```python
from build123d import *

# Parameters (mm, degrees)
F0_W     = 300
F0_H     = 24.5
F0_R     = 2.65
F1_DEPTH = 2
F2_DEPTH = 10
F3_DEPTH = 30
F4_R     = 1.7
F5_DEPTH = 2
F6_R     = 1.25
F7_DEPTH = 2


with BuildPart() as f1:
    # F0 (on Top) → F1 (new body)
    with BuildSketch(Plane.XY):
        Rectangle(F0_W, F0_H)
        with Locations((-60, 0)):
            Circle(F0_R, mode=Mode.SUBTRACT)
        with Locations((-45, 0)):
            Circle(F0_R, mode=Mode.SUBTRACT)
        with Locations((-30, 0)):
            Circle(F0_R, mode=Mode.SUBTRACT)
        with Locations((-15, 0)):
            Circle(F0_R, mode=Mode.SUBTRACT)
        Circle(F0_R, mode=Mode.SUBTRACT)
        with Locations((15, 0)):
            Circle(F0_R, mode=Mode.SUBTRACT)
        with Locations((30, 0)):
            Circle(F0_R, mode=Mode.SUBTRACT)
        with Locations((45, 0)):
            Circle(F0_R, mode=Mode.SUBTRACT)
        with Locations((60, 0)):
            Circle(F0_R, mode=Mode.SUBTRACT)
    extrude(amount=F1_DEPTH)

    # F2 (add): a face of the model
    f2_faces = [f1.faces().sort_by_distance(p)[0] for p in [
        (-150, 0, 1),
    ]]
    extrude(f2_faces, amount=F2_DEPTH)

    # F3 (add): a face of the model
    f3_faces = [f1.faces().sort_by_distance(p)[0] for p in [
        (150, 0, 1),
    ]]
    extrude(f3_faces, amount=F3_DEPTH)

    # F4 (on face) → F5 (cut, through all)
    with BuildSketch(Plane.XY.offset(2)):
        with Locations((-153.6, 0)):
            Circle(F4_R)
    extrude(amount=-F5_DEPTH, mode=Mode.SUBTRACT)

    # F6 (on face) → F7 (cut, through all)
    with BuildSketch(Plane.XY.offset(2)):
        with Locations((158.75, -7.25)):
            Circle(F6_R)
    extrude(amount=-F7_DEPTH, mode=Mode.SUBTRACT)


solid = f1.part
```
Source: CAD feature listing. Evaluate the final solid. Frame: model axes, mm. Coordinates: 2 decimals unless noted, no trailing zeros. Return JSON: item names as keys, results as strings. Group by question number.
1) Contact query for flat-ended pins moving along their axis: P1, Ø3, axis at x = -114, y = 0.5, coming from the -Z side; P2, Ø5, axis at x = -15, y = 0, coming from the -Z side. Output: stop coordinate, or through.
2) Ray query, line 1 along Y through (x, z) = (-153.6, 0.65); line 2 along Y through (x, z) = (0, 1.4); line 3 along X through (y, z) = (-6.25, 0.5). Return the intervals inside material, ascending.
3) Mould query, pull axis X, two halves, no side actions, for faces 1 (the face through (-12.472, 0.796, 0.986)), 2 (the face through (8, 0, 0)). Classes: +X half, -X half, draft (parallel to the pull), parting line (faces both ways), or undercut.
4) Section query A-A, the plane z = 0.3. State how many separate pieces and enclosed holes the cut face has, plus the area to 3 significant figures.
From the geometry:
{
 "1": {"P1": "z = 0", "P2": "through"},
 "2": {"line 1": "-12.25 to -1.7, 1.7 to 12.25", "line 2": "-12.25 to -2.65, 2.65 to 12.25", "line 3": "-160 to 158, 159.5 to 180"},
 "3": {"face 1": "undercut", "face 2": "draft"},
 "4": {"separate pieces": "1", "enclosed holes": "11", "area": "8,120 mm²"}
}
